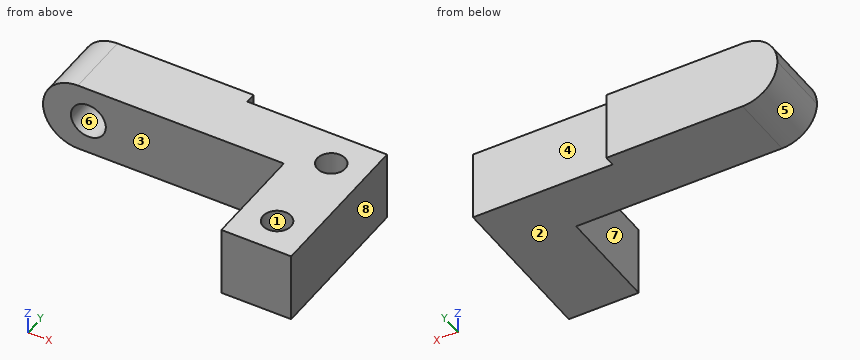
```python
from build123d import *

# Parameters (mm, degrees)
BOSS_EXTRUDE1_DEPTH    = 10
SKETCH2_W              = 20
SKETCH2_H              = 17.246462599
CUT_EXTRUDE1_DEPTH     = 2
FILLET1_R              = 5
SKETCH4_R              = 2.5
CUT_EXTRUDE4_DEPTH     = 5
SKETCH6_W              = 10
SKETCH6_H              = 10
BOSS_EXTRUDE2_DEPTH    = 15
SKETCH5_R              = 2
CUT_EXTRUDE5_DEPTH     = 7
CUT_EXTRUDE6_START     = -0.5
CUT_EXTRUDE6_OUTLINE_W = 25.5
CUT_EXTRUDE6_OUTLINE_H = 12
CUT_EXTRUDE6_DEPTH     = 0.5


# Read off the part's stored shape, not the designer's step: Cut-Extrude6
with BuildPart() as part:
    # Sketch1 → Boss-Extrude1 (new body)
    with BuildSketch(Plane(origin=(0, 0, 0), x_dir=(1, 0, 0), z_dir=(0, 1, 0))):
        Polygon((0, 0), (34.5, 0), (44.5, 0), (44.5, 10), (0, 10), align=None)
    extrude(amount=BOSS_EXTRUDE1_DEPTH)

    # Sketch2 → Cut-Extrude1 (cut)
    with BuildSketch(Plane(origin=(0, 10, 0), x_dir=(1, 0, 0), z_dir=(0, 1, 0))):
        with Locations((34.5, 1.3767687)):
            Rectangle(SKETCH2_W, SKETCH2_H)
    extrude(amount=-CUT_EXTRUDE1_DEPTH, mode=Mode.SUBTRACT)

    # Fillet1
    fillet1_edges = [part.edges().sort_by_distance(p)[0] for p in [
        (0, 5, -10),
        (0, 5, 0),
    ]]
    fillet(fillet1_edges, radius=FILLET1_R - 0.0001)  # a hair under: the kernel refuses the full size

    # Sketch4 → Cut-Extrude4 (cut)
    with BuildSketch(Plane.XZ):
        with Locations(Location((6.5, -5, 0), (0, 0, 270))):
            Circle(SKETCH4_R)
    extrude(amount=-CUT_EXTRUDE4_DEPTH, mode=Mode.SUBTRACT)

    # Sketch6 → Boss-Extrude2 (add)
    with BuildSketch(Plane.XZ):
        with Locations((39.5, -5)):
            Rectangle(SKETCH6_W, SKETCH6_H)
    extrude(amount=BOSS_EXTRUDE2_DEPTH)

    # Sketch5 → Cut-Extrude5 (cut)
    with BuildSketch(Plane.XY):
        with Locations((39.5, 3)):
            Circle(SKETCH5_R)
        with Locations((39.5, -10)):
            Circle(SKETCH5_R)
    extrude(amount=-CUT_EXTRUDE5_DEPTH, mode=Mode.SUBTRACT)

    # Cut-Extrude6 outline → Cut-Extrude6 (cut)
    with BuildSketch(Plane(origin=(0, 10, 0), x_dir=(1, 0, 0), z_dir=(0, 1, 0)).offset(CUT_EXTRUDE6_START)):
        with Locations((11.75, 5)):
            Rectangle(CUT_EXTRUDE6_OUTLINE_W, CUT_EXTRUDE6_OUTLINE_H)
    extrude(amount=CUT_EXTRUDE6_DEPTH, mode=Mode.SUBTRACT)


solid = part.part
```
Input: part model. Units: mm. Frame: model coordinates. Face numbers are marked on the shaded views. A direction names the side the tool comes from. Give positions to 0.01 mm unless a question says otherwise; leave off trailing zeros. Order: outer loops, then holes, each group sorted by start corner. A loop starts at its lowest first (then second) coordinate and runs counter-clockwise, first axis right, second up.
1. Section B-B on z = -2. Return the cut outline in (x, y), and give its area (3 significant figures).
Derived:
outline: (1, 0) - (34.5, 0) - (34.5, -15) - (44.5, -15) - (44.5, 8) - (24.5, 8) - (24.5, 9.5) - (1, 9.5) - close; hole circle Ø4 at (39.5, -10); hole circle Ø4 at (39.5, 3)
area: 508 mm2
2. Material intervals for L1, parallel to Y at x = 39.5, z = -5.25; L2, parallel to X at y = 2.35, z = -5; L3, parallel to Y at x = 29.5, z = -3.75, sorted ascending.
Derived:
L1: y = -15 to -12, -8 to 1, 5 to 8
L2: x = 0 to 4, 9 to 37.61, 41.39 to 44.5
L3: y = 0 to 8
3. Pin query (flat end, axial travel): pin 1 (1.5 mm diameter, centred on x = 17, y = -2.5, fed in from +Z) (3 decimals); pin 2 (5 mm diameter, centred on y = -8, z = -4.5, fed in from -X); pin 3 (2.5 mm diameter, centred on x = 6, z = -6, fed in from -Y); pin 4 (3 mm diameter, centred on x = 39.5, y = 3, fed in from +Z). Return the tip coordinate at first contact, or that it passes through.
Derived:
pin 1: passes through
pin 2: stops at x = 34.5
pin 3: stops at y = 5
pin 4: stops at z = -7
4. Section D-D on y = -10. Return the cut outline in (x, z).
Derived:
outline: (34.5, -10) - (44.5, -10) - (44.5, 0) - (41.5, 0) - (41.5, -7) - (37.5, -7) - (37.5, 0) - (34.5, 0) - close
5. Reachability of the marked faces 1, 2, 3, 4 and 5 from +Z, -Z, +X, -X, +Y, -Y: full face, straight path, thin tool, end or side. Return the list, or none.
Derived:
face 1: +Z
face 2: -Z, +X, -X, +Y, -Y
face 3: +Z, -Z, -X, -Y
face 4: +Z, -Z, +X, +Y
face 5: -Z, -X, +Y, -Y
6. Mould query, pull axis X, two halves, no side actions, for the marked faces 6, 7 and 8. Classes: released by +X, released by -X, zero draft, split by the parting line, or undercut.
Derived:
face 6: undercut
face 7: released by -X
face 8: released by +X
7. Section C-C on x = 39.5. Return the cut outline in (y, z), and give its area (3 significant figures).
Derived:
outline: (-15, -10) - (8, -10) - (8, 0) - (5, 0) - (5, -7) - (1, -7) - (1, 0) - (-8, 0) - (-8, -7) - (-12, -7) - (-12, 0) - (-15, 0) - close
area: 174 mm2
